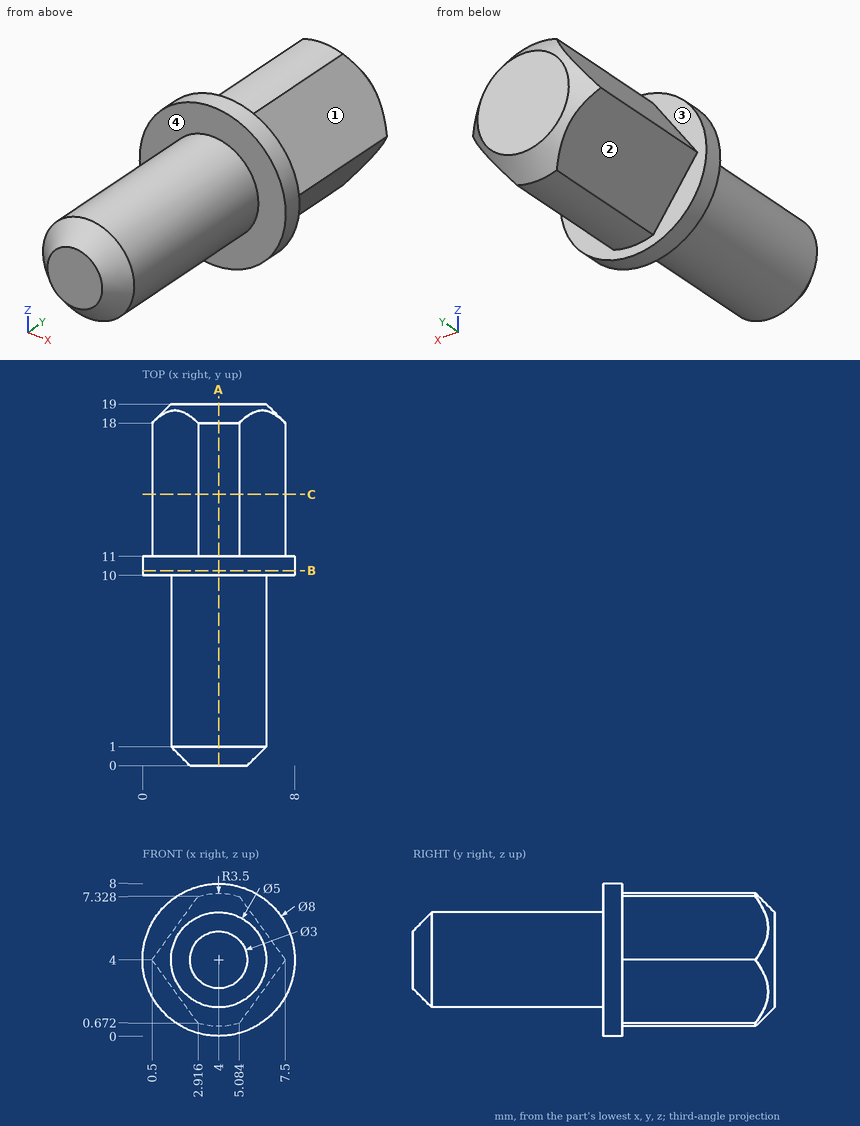
The drawing under review shows one solid part. Ordinate dimensions are in mm from its lowest x, y, z. A direction names the side the tool comes from. Coordinates: 2 decimals unless noted, no trailing zeros. Order: outer loops, then holes, each group sorted by start corner. A loop starts at its lowest first (then second) coordinate and runs counter-clockwise, first axis right, second up. Notation, with made-up numbers: M 75.25,76 L 89.25,76 A18 ccw 89.25,110 Z; hole C -4.5,9.25 d3. An arc over 180 degrees is marked long. Use a Markdown table: item, result.
(1) For P1, Ø1, axis at y = 15.5, z = 5, coming from the +X side; P2, Ø4, axis at x = 2, y = 7.5, coming from the -Z side; P3, Ø4, axis at x = 6.5, y = 3, coming from the +Z side, all flat-tipped, find the tip position at first contact; note any pin that passes through.
Worked answers:
| item | result |
|---|---|
| P1 | stops at x = 7.14 |
| P2 | stops at z = 1.5 |
| P3 | stops at z = 6.45 |
(2) Add section A-A (x = 4). Give the boundary of the cut face in (y, z).
Worked answers:
| item | result |
|---|---|
| outline | M 0,2.5 L 1,1.5 L 10,1.5 L 10,0 L 11,0 L 11,0.5 L 18,0.5 L 19,1.5 L 19,6.5 L 18,7.5 L 11,7.5 L 11,8 L 10,8 L 10,6.5 L 1,6.5 L 0,5.5 Z |
(3) Add section B-B (y = 10.25). Give the boundary of the cut face in (x, z), then the cut area to 3 significant figures.
Worked answers:
| item | result |
|---|---|
| outline | C 4,4 d8 |
| area | 50.3 mm2 |
(4) For the marked faces 1, 2, 3 and 4, list the 3-axis set-ups (+Z, -Z, +X, -X, +Y, -Y) from which the entire face can be reached by the end or side of a thin tool; tool diameter is ignored.
Worked answers:
| item | result |
|---|---|
| face 1 | +Z, +X, +Y |
| face 2 | -Z, -X, +Y |
| face 3 | +Y |
| face 4 | -Y |
(5) Wall thickness on probe 1 along Y at (x, z) = (6.75, 5.25); probe 2 along Z at (x, y) = (0.75, 15.25) (1 decimal); probe 3 along Y at (x, z) = (2.75, 2.25): over which ranges is each line inside the solid? List them lowest first.
Worked answers:
| item | result |
|---|---|
| probe 1 | y = 10 to 11 |
| probe 2 | z = 3.7 to 4.3 |
| probe 3 | y = 0.65 to 19 |
(6) Add section C-C (y = 14.25). Give the boundary of the cut face in (x, z).
Worked answers:
| item | result |
|---|---|
| outline | M 0.5,4 L 2.92,0.67 A3.5 ccw 5.08,0.67 L 7.5,4 L 5.08,7.33 A3.5 ccw 2.92,7.33 Z |
